Design review of the part built by this model. Coordinates are the model's own, in mm. Coordinates: 2 decimals unless noted, no trailing zeros. Write each loop counter-clockwise with the first axis right and the second up, starting at its lowest first coordinate (ties: lowest second). Pieces come first, ordered by that corner, then holes. Notation, with made-up numbers: (13.5, -12) -> (55.5, -12) arc R11 cw to (55.5, 2) -> close; hole circle Ø6 at (67.5, -20.5). An arc over 180 degrees is marked (long way). Return JSON: item names as keys, results as strings. Group by question number.
from build123d import *

# Parameters (mm, degrees)
F1_DEPTH = 3.175


with BuildPart() as f1:
    # F0 (on Top) → F1 (new body)
    with BuildSketch(Plane.XY):
        with BuildLine():
            Line((0, 0), (0, 231.775))
            Line((0, 231.775), (-44.45, 231.775))
            ThreePointArc((-44.45, 231.775), (-134.252561, 194.577561), (-171.45, 104.775))
            Line((-171.45, 104.775), (-171.45, 0))
            Line((-171.45, 0), (0, 0))
        make_face()
        with BuildLine():
            Line((44.581378, 231.775), (0, 231.775))
            Line((0, 231.775), (0, 0))
            Line((0, 0), (171.45, 0))
            Line((171.45, 0), (171.581278, 104.615633))
            ThreePointArc((171.581278, 104.615633), (134.440266, 194.521199), (44.581378, 231.775))
        make_face()
        with BuildLine():
            Line((171.45, 0), (0, 0))
            Line((0, 0), (0, -231.775))
            Line((0, -231.775), (44.243227, -231.847034))
            ThreePointArc((44.243227, -231.847034), (134.179426, -194.722839), (171.45, -104.847202))
            Line((171.45, -104.847202), (171.45, 0))
        make_face()
        with BuildLine():
            Line((0, -231.775), (0, 0))
            Line((0, 0), (-171.45, 0))
            Line((-171.45, 0), (-171.45, -104.775))
            ThreePointArc((-171.45, -104.775), (-134.252561, -194.577561), (-44.45, -231.775))
            Line((-44.45, -231.775), (0, -231.775))
        make_face()
    extrude(amount=F1_DEPTH)


solid = f1.part
Q1. We need section C-C on x = 129. Write out the cut boundary in (y, z) (3 decimals), plus the area to 3 significant figures.
Q2. We need section A-A on z = 2.6. Write out the cut boundary in (x, y) (3 decimals).
Q3. We need section B-B on y = 195. Write out the cut boundary in (x, z) (1 decimal), plus the area to 3 significant figures.
Q4. Wall thickness on L1, parallel to X at y = -57.5, z = 0.4; L2, parallel to X at y = 24, z = 2; L3, parallel to Y at x = 2, z = 1.6 (3 decimals): over which ranges is each line inside the solid? List them lowest first.
Q5. For P1, Ø1.6, axis at y = -54.5, z = 1, coming from the +X side, flat-tipped, find the tip position at first contact; note if it passes through.
Findings below:
{
 "1": {"outline": "(-199.612, 0) -> (199.656, 0) -> (199.656, 3.175) -> (-199.612, 3.175) -> close", "area": "1,270 mm^2"},
 "2": {"outline": "(-171.45, -104.775) arc R127 ccw to (-44.45, -231.775) -> (0, -231.775) -> (44.243, -231.847) arc R127 ccw to (171.45, -104.847) -> (171.45, 0) -> (171.581, 104.616) arc R127 ccw to (44.581, 231.775) -> (-44.45, 231.775) arc R127 ccw to (-171.45, 104.775) -> close"},
 "3": {"outline": "(-133.8, 0) -> (134, 0) -> (134, 3.2) -> (-133.8, 3.2) -> close", "area": "850 mm^2"},
 "4": {"L1": "x = -171.45 to 171.45", "L2": "x = -171.45 to 171.48", "L3": "y = -231.778 to 231.775"},
 "5": {"P1": "stops at x = 171.45"}
}
